CAD build for the part. Positions are in the model's coordinates, mm. Face numbers are marked on the shaded views. Give positions to 0.01 mm unless a question says otherwise; leave off trailing zeros. Write each loop counter-clockwise with the first axis right and the second up, starting at its lowest first coordinate (ties: lowest second). Pieces come first, ordered by that corner, then holes. Notation, with made-up numbers: (-30.5, 75) -> (24.5, 75) arc R31 cw to (24.5, 107) -> close; hole circle Ø2 at (-33.75, -16). An arc over 180 degrees is marked (long way). Answer as a JSON object with one key per item and string values.
Autodesk Inventor part; units mm, degrees
ref_plane "YZ Plane" through (0, 0, 0) normal (1, 0, 0) x (0, 1, 0)
ref_plane "XZ Plane" through (0, 0, 0) normal (0, 1, 0) x (-1, 0, 0)
ref_plane "XY Plane" through (0, 0, 0) normal (0, 0, 1) x (1, 0, 0)
sketch "Sketch1" plane through (0, 0, 0) normal (0, 0, 1) x (1, 0, 0)
  line L0 (-4.4434, -31.1874) -> (-7.8728, -29.4435)
  arc A0 (4.4434, -31.1874) -> (-4.4434, -31.1874) centre (0, -41.25) ccw
  line L1 (7.8728, -29.4435) -> (4.4434, -31.1874)
  line L2 (7.8728, -29.4435) -> (9.9951, 38.4375)
  arc A1 (9.9951, 38.4375) -> (-9.9951, 38.4375) centre (0, 38.75) ccw
  line L3 (-9.9951, 38.4375) -> (-7.8728, -29.4435)
  circle A2 centre (0, -26.25) radius 1.5
  circle A3 centre (0, -16.25) radius 1.5
  circle A4 centre (0, -41.25) radius 7.5
  line L4 (0, -16.25) -> (0, -9.25)
  line L5 (0, -9.25) -> (8.4958, -9.5156)
  line L6 (0, -9.25) -> (-8.4958, -9.5156)
  line L7 (0, -41.25) -> (7.4963, -41.4844)
  line L8 (0, -41.25) -> (-7.4963, -41.4844)
  line L9 (-8.4958, -9.5156) -> (-7.4963, -41.4844)
  line L10 (7.4963, -41.4844) -> (8.4958, -9.5156)
  arc A5 (-7.4963, -41.4844) -> (7.4963, -41.4844) centre (0, -41.25) ccw
  point P0 (0, 0)
  dimension "d0" = 15
  dimension "d1" = 7
  dimension "d2" = 7.5
extrude "Extrusion1" add sketch "Sketch1" along normal blind 5 contours A0 L1 L10 A4 L9 L0 | L0 L3 L6 L5 L2 L1 A0 | L8 L7 A4 | A4 L7 L8
chamfer "Chamfer1" distance 2 angle 45 3 edges at (-8.1843, -19.4796, 5) (0, -48.75, 5) (8.1843, -19.4796, 5)
fillet "Fillet1" radius 60 1 edges at (0, -9.25, 2.5)
properties part number "leg_bone_2"
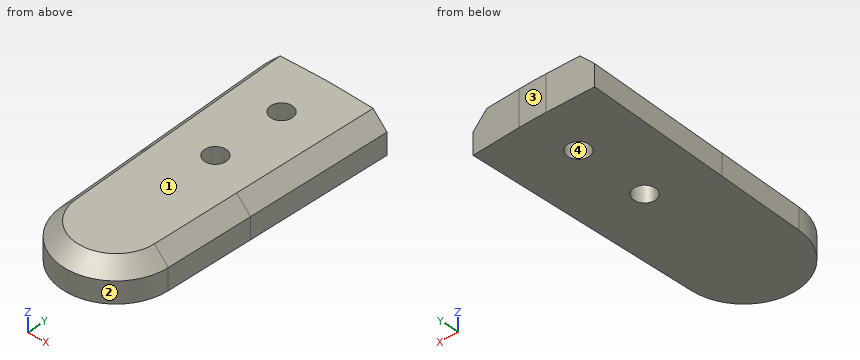
1) Slice it at B-B (y = -16.25). List the corners of the cut face in (x, z).
Model answer:
{"outline": "(-8.29, 0) -> (-1.5, 0) -> (-1.5, 5) -> (-6.28, 5) -> (-8.29, 3) -> close; (1.5, 0) -> (8.29, 0) -> (8.29, 3) -> (6.28, 5) -> (1.5, 5) -> close"}
2) Slice it at C-C (z = 4.4). List the corners of the cut face in (x, y), then the cut area to 3 significant figures.
Model answer:
{"outline": "(-7.1, -9.47) -> (-6.47, -29.4) -> (-6.1, -41.44) arc R6.1 ccw to (6.1, -41.44) -> (6.47, -29.4) -> (7.1, -9.47) -> (1.87, -9.31) arc R60 ccw to (-1.87, -9.31) -> close; hole circle Ø3 at (0, -26.25); hole circle Ø3 at (0, -16.25)", "area": "465 mm2"}
3) Slice it at D-D (y = -38.5). List the corners of the cut face in (x, z), then the cut area to 3 significant figures.
Model answer:
{"outline": "(-7.59, 0) -> (7.59, 0) -> (7.59, 3) -> (5.59, 5) -> (-5.59, 5) -> (-7.59, 3) -> close", "area": "71.9 mm2"}
4) Pin check, flat tips, straight feed: pin 1 (1 mm diameter, centred on x = -1.5, z = 2, fed in from -Y); pin 2 (1.5 mm diameter, centred on x = 6.5, z = 2.5, fed in from -Y); pin 3 (2.5 mm diameter, centred on x = 0, y = -26.25, fed in from +Z); pin 4 (3 mm diameter, centred on y = -41, z = 3, fed in from +X). Stop position of each tip, or through.
Model answer:
{"pin 1": "stops at y = -48.68", "pin 2": "stops at y = -46.07", "pin 3": "passes through", "pin 4": "stops at x = 7.56"}
5) Wall check: probe 1 along Y at (x, z) = (0, 1.35); probe 2 along Y at (x, z) = (0, 3.15); probe 3 along X at (y, z) = (-18, 0.85). Give the ranges that are in metal, low to high.
Model answer:
{"probe 1": "y = -48.75 to -27.75, -24.75 to -17.75, -14.75 to -9.28", "probe 2": "y = -48.6 to -27.75, -24.75 to -17.75, -14.75 to -9.28", "probe 3": "x = -8.23 to 8.23"}
6) Mould opens along Y. For the marked faces 1, 2, 3 and 4 say: released by +Y, released by -Y, zero draft, split by the parting line, or undercut.
Model answer:
{"face 1": "zero draft", "face 2": "released by -Y", "face 3": "released by +Y", "face 4": "undercut"}
7) Slice it at A-A (x = 0). List the corners of the cut face in (y, z).
Model answer:
{"outline": "(-48.75, 0) -> (-27.75, 0) -> (-27.75, 5) -> (-46.75, 5) -> (-48.75, 3) -> close; (-24.75, 0) -> (-17.75, 0) -> (-17.75, 5) -> (-24.75, 5) -> close; (-14.75, 0) -> (-9.28, 0) -> (-9.28, 5) -> (-14.75, 5) -> close"}
